Autodesk Inventor part; units mm, degrees
ref_plane "YZ Plane" through (0, 0, 0) normal (1, 0, 0) x (0, 1, 0)
ref_plane "XZ Plane" through (0, 0, 0) normal (0, 1, 0) x (-1, 0, 0)
ref_plane "XY Plane" through (0, 0, 0) normal (0, 0, 1) x (1, 0, 0)
sketch "Boceto1" plane through (0, 0, 0) normal (0, 1, 0) x (-1, 0, 0)
  circle A0 centre (0, 0) radius 9.1
  dimension "d0" = 18.2
extrude "Extrusión1" add sketch "Boceto1" along normal blind 20
sketch "Boceto2" plane through (0, 20, 0) normal (0, 1, 0) x (1, 0, 0)
  circle A0 centre (0, 0) radius 5
  dimension "d3" = 10
extrude "Extrusión2" add sketch "Boceto2" along normal blind 14
sketch "Boceto3" plane through (0, 34, 0) normal (0, 1, 0) x (1, 0, 0)
  circle A0 centre (0, 0) radius 5
hole "Agujero1" at (0, 34, 0) direction (0, -1, 0) diameter 7 end through all
chamfer "Chaflán1" distance 2 angle 45 1 edges at (9.1, 0, 0)
chamfer "Chaflán2" distance 1 angle 45 1 edges at (-5, 34, 0)
thread "Rosca1"
properties part number "Acople E27"
Build history of the part. All positions in model axes, mm. A direction names the side the tool comes from. Give positions to 0.01 mm unless a question says otherwise; leave off trailing zeros. Loops run counter-clockwise (first coordinate to the right, second up) from the corner with the lowest first, then second, coordinate; pieces in that order, holes last.
Item 1: Pull direction X, two halves, no side cores. Call faces 3 (the face through (-6.891, 0.125, 2.17)), 4 (the face through (1.341, 16.762, 3.233)), 5 (the face through (-4, 20, -4)): released by +X, released by -X, zero draft, split by the parting line, or undercut.
Answers follow:
face 3: split by the parting line
face 4: undercut
face 5: zero draft
Item 2: Which spindle directions (+Z, -Z, +X, -X, +Y, -Y) get a long thin tool onto all of the face, cutting with end or side? Do faces 1 (the face through (3.3, 0, 1.7)), 2 (the face through (-1.08, 26.41, -4.88)). Say none if no direction does.
Answers follow:
face 1: +Z, -Z, +X, -X, -Y
face 2: +Y
Item 3: Flat gauge pins, fed straight in: pin 1 (5 mm diameter, centred on x = -4.5, y = 22, fed in from -Z); pin 2 (1 mm diameter, centred on x = -2.5, y = 9.5, fed in from +Z); pin 3 (6 mm diameter, centred on y = 18, z = -5.5, fed in from +X). Where does each tip first touch, or does it go through?
Answers follow:
pin 1: stops at z = -8.59
pin 2: stops at z = 8.88
pin 3: stops at x = 8.75
Item 4: Slice it at C-C, the plane y = 23. List the corners of the cut face in (x, z).
Answers follow:
outline: circle Ø10 at (0, 0); hole circle Ø7 at (0, 0)
Item 5: Slice it at A-A, the plane z = 0. List the corners of the cut face in (x, y), and give its area (3 significant figures).
Answers follow:
outline: (-9.1, 2) - (-7.1, 0) - (-3.5, 0) - (-3.5, 34) - (-4, 34) - (-5, 33) - (-5, 20) - (-9.1, 20) - close; (3.5, 0) - (7.1, 0) - (9.1, 2) - (9.1, 20) - (5, 20) - (5, 33) - (4, 34) - (3.5, 34) - close
area: 261 mm2
Item 6: Slice it at B-B, the plane x = 0. List the corners of the cut face in (y, z).
Answers follow:
outline: (0, -7.1) - (2, -9.1) - (20, -9.1) - (20, -5) - (33, -5) - (34, -4) - (34, -3.5) - (0, -3.5) - close; (0, 3.5) - (34, 3.5) - (34, 4) - (33, 5) - (20, 5) - (20, 9.1) - (2, 9.1) - (0, 7.1) - close
Item 7: Drill centre lines: line 1 (Z direction, x = 0, y = 11); line 2 (X direction, y = 29.5, z = 0.25); line 3 (Y direction, x = 4, z = -4.25). Where is each one in solid material? Low to high.
Answers follow:
line 1: z = -9.1 to -3.5, 3.5 to 9.1
line 2: x = -4.99 to -3.49, 3.49 to 4.99
line 3: y = 0 to 20
Item 8: Slice it at D-D, the plane y = 8. List the corners of the cut face in (x, z), and give its area (3 significant figures).
Answers follow:
outline: circle Ø18.2 at (0, 0); hole circle Ø7 at (0, 0)
area: 222 mm2
